Source: CAD feature listing. Evaluate the final solid. Frame: model axes, mm. Round coordinates to 2 decimals unless told otherwise and drop trailing zeros. Order: outer loops, then holes, each group sorted by start corner. A loop starts at its lowest first (then second) coordinate and runs counter-clockwise, first axis right, second up. Notation, with made-up numbers: (17.5, 10.25) - (73.5, 10.25) arc R33 cw to (73.5, 41.25) - close; hole circle Ø1 at (-8, 45.5). An arc over 180 degrees is marked (long way). Return JSON: item names as keys, results as strings. Group by question number.
1) Contact query for flat-ended pins moving along their axis: P1, Ø10, axis at x = 2.5, z = 83.5, coming from the -Y side; P2, Ø12, axis at y = 5, z = 66.5, coming from the +X side; P3, Ø3, axis at y = 0.5, z = 47.5, coming from the -X side. Output: stop coordinate, or through.
2) Section A-A, the plane y = 0. Return loops of the section in (x, z), plus the area to 3 significant figures.
3) Section D-D, the plane z = 40.5. Return loops of the section in (x, y).
4) Section B-B, the plane x = 0. Return loops of the section in (y, z).
5) Ray query, line 1 (X direction, y = 0, z = -2.5); line 2 (X direction, y = 0, z = 5.5); line 3 (Z direction, x = -5, y = 2). Return the intervals inside material, ascending. Write a range as from..to.
6) Section C-C, the plane z = 0. Return loops of the section in (x, y).
```python
from build123d import *

# Parameters (mm, degrees)
F0_R     = 10
F0_R_2   = 4
F1_DEPTH = 25
F2_R     = 2
F3_DEPTH = 12.5
F5_START = 12.5
F4_R     = 4
F5_DEPTH = 2
F7_START = 15
F6_R     = 4
F7_DEPTH = 85


with BuildPart() as f1:
    # F0 (on Top) → F1 (new body, symmetric)
    with BuildSketch(Plane.XY):
        Circle(F0_R)
        Circle(F0_R_2, mode=Mode.SUBTRACT)
    extrude(amount=F1_DEPTH, both=True)

    # F2 (on Right) → F3 (join, symmetric)
    with BuildSketch(Plane.YZ):
        Circle(F2_R)
    extrude(amount=F3_DEPTH, both=True)

    # F4 (on Right) → F5 (join)
    with BuildSketch(Plane.YZ.offset(F5_START)):
        Circle(F4_R)
    extrude(amount=F5_DEPTH)

    # F6 (on Top) → F7 (join)
    with BuildSketch(Plane.XY.offset(F7_START)):
        Circle(F6_R)
    extrude(amount=F7_DEPTH)


solid = f1.part
```
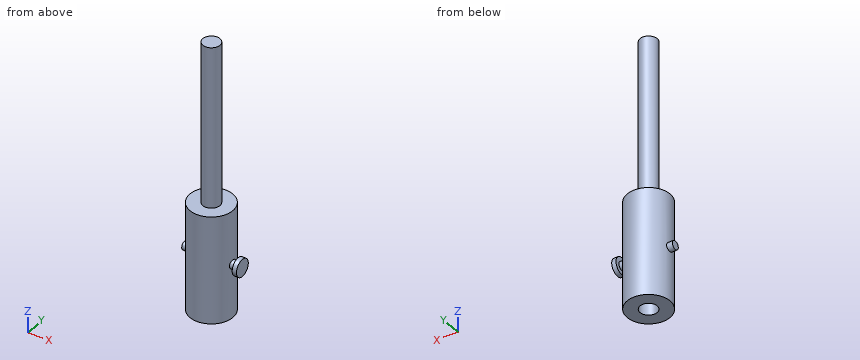
Geometry check:
{
 "1": {"P1": "y = -4", "P2": "x = 4", "P3": "x = -4"},
 "2": {"outline": "(-12.5, -2) - (-10, -2) - (-10, -25) - (-4, -25) - (-4, -2) - (4, -2) - (4, -25) - (10, -25) - (10, -2) - (12.5, -2) - (12.5, -4) - (14.5, -4) - (14.5, 4) - (12.5, 4) - (12.5, 2) - (10, 2) - (10, 25) - (4, 25) - (4, 100) - (-4, 100) - (-4, 25) - (-10, 25) - (-10, 2) - (-12.5, 2) - close; hole (-4, 2) - (4, 2) - (4, 15) - (-4, 15) - close", "area": "1,350 mm2"},
 "3": {"outline": "circle Ø8 at (0, 0)"},
 "4": {"outline": "(-10, -25) - (-4, -25) - (-4, 15) - (4, 15) - (4, -25) - (10, -25) - (10, 25) - (4, 25) - (4, 100) - (-4, 100) - (-4, 25) - (-10, 25) - close; circle Ø4 at (0, 0)"},
 "5": {"line 1": "-10..-4, 4..10, 12.5..14.5", "line 2": "-10..-4, 4..10", "line 3": "-25..25"},
 "6": {"outline": "(-12.5, -2) - (-9.8, -2) arc R10 ccw to (9.8, -2) - (12.5, -2) - (12.5, -4) - (14.5, -4) - (14.5, 4) - (12.5, 4) - (12.5, 2) - (9.8, 2) arc R10 ccw to (-9.8, 2) - (-12.5, 2) - close; hole (-3.46, -2) arc R4 ccw to (3.46, -2) - close; hole (-3.46, 2) - (3.46, 2) arc R4 ccw to start"}
}
